from build123d import *

# Parameters (mm, degrees)
SKETCH1_R           = 1.5
SKETCH1_W           = 27.94
SKETCH1_H           = 5.842
BOSS_EXTRUDE1_DEPTH = 3.81
SKETCH2_W           = 5.588
SKETCH2_H           = 5.842
CUT_EXTRUDE1_DEPTH  = 1.2


with BuildPart() as part:
    # Sketch1 → Boss-Extrude1 (new body)
    # profile 1 of 3: a face of its own
    with BuildSketch(Plane.XY):
        Polygon((-13.97, -3.81), (-13.97, -2.921), (-13.97, 2.921), (-13.97, 3.81), (-21.59, 3.81), (-21.59, -3.81), align=None)
        with Locations(Location((-17.78, 0, 0), (0, 0, 180))):
            Circle(SKETCH1_R, mode=Mode.SUBTRACT)
    # profile 2 of 3: a face of its own
    with BuildSketch(Plane.XY):
        Rectangle(SKETCH1_W, SKETCH1_H)
    # profile 3 of 3: a face of its own
    with BuildSketch(Plane.XY):
        Polygon((13.97, 2.921), (13.97, -2.921), (13.97, -3.81), (21.59, -3.81), (21.59, 3.81), (13.97, 3.81), align=None)
        with Locations(Location((17.78, 0, 0), (0, 0, 180))):
            Circle(SKETCH1_R, mode=Mode.SUBTRACT)
    extrude(amount=BOSS_EXTRUDE1_DEPTH)

    # Sketch2 → Cut-Extrude1 (cut)
    with BuildSketch(Plane.XY.offset(3.81)):
        Rectangle(SKETCH2_W, SKETCH2_H)
    extrude(amount=-CUT_EXTRUDE1_DEPTH, mode=Mode.SUBTRACT)


solid = part.part
The listing builds one solid part. Answer for the finished solid, in the listing's coordinates (mm). A direction names the side the tool comes from. Give positions to 0.01 mm unless a question says otherwise; leave off trailing zeros. Order: outer loops, then holes, each group sorted by start corner. A loop starts at its lowest first (then second) coordinate and runs counter-clockwise, first axis right, second up. Notation, with made-up numbers: (86.5, 48.25) - (119.5, 48.25) arc R13 ccw to (119.5, 52.25) - close; hole circle Ø7 at (68, 59.5). An arc over 180 degrees is marked (long way). One line per item, written item: value. Start each with the question number.
1) A cutting plane is placed at C-C on z = 1.4. Give the vertices of the cut face in (x, y).
2) A cutting plane is placed at A-A on y = 0. Give the vertices of the cut face in (x, z).
3) A cutting plane is placed at B-B on x = 17.78. Give the vertices of the cut face in (y, z), then the cut area to 3 significant figures.
4) A cutting plane is placed at D-D on x = -7. Give the vertices of the cut face in (y, z).
5) A tool of negligible diameter and unlimited length cuts with its end or side. For faces 4 (the face through (13.97, 3.4, 1.9)), 5 (the face through (-19.21, -0.45, 1.88)), 6 (the face through (2.794, 0, 3)), 7 (the face through (18, 3.81, 2)), 8 (the face through (-13.97, -3.4, 1.9)), from which of +Z, -Z, +X, -X, +Y, -Y can it reach the whole face along a straight path? Write none if from no direction.
6) Find the intervals of material crossed by L1, parallel to Y at x = -17.78, z = 1.7; L2, parallel to X at y = -0.5, z = 2.9; L3, parallel to Y at x = 7, z = 3.1, in increasing order.
7) Given pin 1 Ø1.1 at (x, z) = (-3, 1.5) entering from -Y, flat-ended and moving along its own axis, determine where the tip first touches the part or whether it passes through.
8) The mould has two halves that part along X. Classify faces 1 (the face through (0, 0, 2.61)), 2 (the face through (0, 0, 0)), 3 (the face through (-21.59, 0, 2)): released by +X, released by -X, zero draft, split by the parting line, or undercut.
Answer sheet:
1. outline: (-21.59, -3.81) - (-13.97, -3.81) - (-13.97, -2.92) - (13.97, -2.92) - (13.97, -3.81) - (21.59, -3.81) - (21.59, 3.81) - (13.97, 3.81) - (13.97, 2.92) - (-13.97, 2.92) - (-13.97, 3.81) - (-21.59, 3.81) - close; hole circle Ø3 at (-17.78, 0); hole circle Ø3 at (17.78, 0)
2. outline: (-21.59, 0) - (-19.28, 0) - (-19.28, 3.81) - (-21.59, 3.81) - close; (-16.28, 0) - (16.28, 0) - (16.28, 3.81) - (2.79, 3.81) - (2.79, 2.61) - (-2.79, 2.61) - (-2.79, 3.81) - (-16.28, 3.81) - close; (19.28, 0) - (21.59, 0) - (21.59, 3.81) - (19.28, 3.81) - close
3. outline: (-3.81, 0) - (-1.5, 0) - (-1.5, 3.81) - (-3.81, 3.81) - close; (1.5, 0) - (3.81, 0) - (3.81, 3.81) - (1.5, 3.81) - close
3. area: 17.6 mm2
4. outline: (-2.92, 0) - (2.92, 0) - (2.92, 3.81) - (-2.92, 3.81) - close
5. face 4: +Z, -Z, +Y
5. face 5: +Z, -Z
5. face 6: +Z, +Y, -Y
5. face 7: +Z, -Z, +X, -X, +Y
5. face 8: +Z, -Z, -Y
6. L1: y = -3.81 to -1.5, 1.5 to 3.81
6. L2: x = -21.59 to -19.19, -16.37 to -2.79, 2.79 to 16.37, 19.19 to 21.59
6. L3: y = -2.92 to 2.92
7. pin 1: stops at y = -2.92
8. face 1: undercut
8. face 2: zero draft
8. face 3: released by -X
